Autodesk Inventor part; units mm, degrees
ref_plane "YZ Plane" through (0, 0, 0) normal (1, 0, 0) x (0, 1, 0)
ref_plane "XZ Plane" through (0, 0, 0) normal (0, 1, 0) x (-1, 0, 0)
ref_plane "XY Plane" through (0, 0, 0) normal (0, 0, 1) x (1, 0, 0)
sketch "Sketch1" plane through (0, 0, 0) normal (0, 0, 1) x (1, 0, 0)
  line L0 (-20.1009, 13.5086) -> (29.8991, 13.5086)
  line L1 (29.8991, 13.5086) -> (29.8991, -18.4914)
  line L2 (29.8991, -18.4914) -> (-20.1009, -18.4914)
  line L3 (-20.1009, -18.4914) -> (-20.1009, 13.5086)
  point P0 (0, 0)
  dimension "d0" = 50
  dimension "d1" = 32
extrude "Extrusion1" add sketch "Sketch1" along normal blind 40
sketch "Sketch2" plane through (0, 0, 40) normal (0, 0, 1) x (1, 0, 0)
  line L0 (-20.1009, -18.4914) -> (-20.1009, 13.5086)
  line L1 (29.8991, -18.4914) -> (-20.1009, -18.4914)
  line L2 (-20.1009, -2.4914) -> (-8.6009, -2.4914)
  circle A0 centre (-8.6009, -2.4914) radius 8
  point P0 (0, 0)
  dimension "d4" = 11.5
  dimension "d5" = 16
extrude "Extrusion2" cut sketch "Sketch2" against normal blind 10
sketch "Sketch3" plane through (0, 0, 40) normal (0, 0, 1) x (1, 0, 0)
  circle A0 centre (-8.6009, -2.4914) radius 8
  point P0 (0, 0)
extrude "Extrusion3" add sketch "Sketch3" against normal blind 10
sketch "Sketch4" plane through (0, 0, 40) normal (0, 0, 1) x (1, 0, 0)
  line L0 (-20.1009, -18.4914) -> (-20.1009, 13.5086)
  line L1 (29.8991, -18.4914) -> (-20.1009, -18.4914)
  line L2 (-20.1009, -2.4914) -> (-8.6009, -2.4914)
  circle A0 centre (-8.6009, -2.4914) radius 11
  point P0 (0, 0)
  dimension "d10" = 11.5
  dimension "d11" = 22
extrude "Extrusion4" cut sketch "Sketch4" against normal blind 10
properties part number "basic1"
Work out the finished part from the listing and answer in its coordinate system (mm). A direction names the side the tool comes from. Round coordinates to 2 decimals unless told otherwise and drop trailing zeros. Write each loop counter-clockwise with the first axis right and the second up, starting at its lowest first coordinate (ties: lowest second). Pieces come first, ordered by that corner, then holes. Notation, with made-up numbers: (-8.75, 23) - (43.25, 23) arc R33 ccw to (43.25, 60) - close; hole circle Ø1 at (68.5, 11.5). An arc over 180 degrees is marked (long way). Answer in a Markdown table with one row per item. Add a question column.
1. Given pin 1 (6.5 mm diameter, centred on x = -8.5, y = -7.5, fed in from +Z), flat-ended and moving along its own axis, determine where the tip first touches the part or whether it passes through.
2. A cutting plane is placed at C-C, the plane z = 32. Determine the outline of the cut face in (x, y).
3. For faces 1 (the flat face through (-9, -2, 30)), 2 (the flat face through (10, -2, 40)), determine the directions among +Z, -Z, +X, -X, +Y, -Y from which every point of the face is accessible in a straight line to the end or side of a thin tool.
4. The mould has two halves that part along Y. Classify faces 3 (the cylindrical face through (1.89, 0.81, 35.07)), 4 (the flat face through (5, 13.509, 20)), 5 (the flat face through (5, -18.491, 20)), 6 (the flat face through (-20.101, -3, 20)): +Y half, -Y half, draft (parallel to the pull), parting line (faces both ways), or undercut.
5. A cutting plane is placed at B-B, the plane y = -6. Determine the outline of the cut face in (x, z), and give its area (3 significant figures).
6. A cutting plane is placed at A-A, the plane x = -2.5. Determine the outline of the cut face in (y, z), and give its area (3 significant figures).
7. Find the intervals of material crossed by line 1 along Z through (x, y) = (-10.5, -10.5); line 2 along X through (y, z) = (-6.5, 36.5); line 3 along Y through (x, z) = (-3, 36.5), in increasing order. Write a range as from..to.
Worked out:
| question | item | result |
|---|---|---|
| 1 | pin 1 | z = 30 |
| 2 | outline | (-20.1, -18.49) - (29.9, -18.49) - (29.9, 13.51) - (-20.1, 13.51) - close; hole circle Ø22 at (-8.6, -2.49) |
| 3 | face 1 | +Z |
| 3 | face 2 | +Z, +X, -X, +Y, -Y |
| 4 | face 3 | undercut |
| 4 | face 4 | +Y half |
| 4 | face 5 | -Y half |
| 4 | face 6 | draft |
| 5 | outline | (-20.1, 0) - (29.9, 0) - (29.9, 40) - (1.82, 40) - (1.82, 30) - (-19.03, 30) - (-19.03, 40) - (-20.1, 40) - close |
| 5 | area | 1,790 mm^2 |
| 6 | outline | (-18.49, 0) - (13.51, 0) - (13.51, 40) - (6.66, 40) - (6.66, 30) - (-11.64, 30) - (-11.64, 40) - (-18.49, 40) - close |
| 6 | area | 1,100 mm^2 |
| 7 | line 1 | 0..30 |
| 7 | line 2 | -20.1..-18.84, 1.64..29.9 |
| 7 | line 3 | -18.49..-11.96, 6.98..13.51 |
